Read the model definition and answer for the solid it produces. Units are mm, in the model's axes. Face numbers are marked on the shaded views. A direction names the side the tool comes from. Coordinates: 2 decimals unless noted, no trailing zeros. Order: outer loops, then holes, each group sorted by start corner. A loop starts at its lowest first (then second) coordinate and runs counter-clockwise, first axis right, second up.
Autodesk Fusion 360 part; units mm, degrees
box "BoxPrimitive1" add length 65 width 15 height 4 placed x (0, 0, -1) y (-1, 0, 0) z (0, 1, 0) at (0, 0, 0)
sketch "Sketch2" plane through (0, 4, 0) normal (0, 1, 0) x (-1, 0, 0)
  line L0 (0, -65) -> (15, -65)
  line L1 (15, -65) -> (15, 0)
  line L2 (15, 0) -> (0, 0)
  line L3 (0, 0) -> (0, -65)
  line L4 (15, -65) -> (0, -65)
  line L5 (0, -65) -> (0, -61)
  line L6 (0, -61) -> (15, -61)
  line L7 (15, -61) -> (15, -65)
  dimension "d6" = 4
extrude "Extrude1" add sketch "Sketch2" along normal blind 35 contours L0 L1 L3 L4 L5 L6 L7
chamfer "Chamfer1" distance 9 angle 45 1 edges at (-7.5, 4, -61)
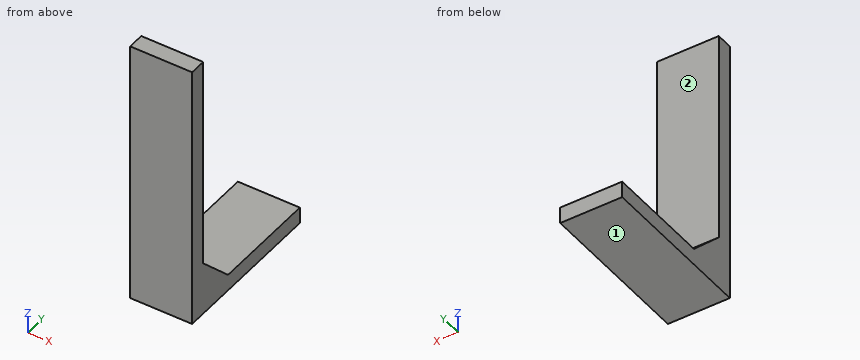
1) A cutting plane is placed at C-C, the plane y = 6.5. Determine the outline of the cut face in (x, z), and give its area (4 significant figures).
A:
outline: (-15, -65) - (0, -65) - (0, -54.5) - (-15, -54.5) - close
area: 157.5 mm2
2) Straight lines are drawn through the part: line 1 (Y direction, x = -7.75, z = -44.5); line 2 (Z direction, x = -11, y = 36.5); line 3 (Y direction, x = -7.75, z = -60). For each, find the intervals that lie inside material, in ascending order.
A:
line 1: y = 0 to 4
line 2: z = -65 to -61
line 3: y = 0 to 12
3) A cutting plane is placed at A-A, the plane x = -3.5. Determine the outline of the cut face in (y, z), and give its area (4 significant figures).
A:
outline: (0, -65) - (39, -65) - (39, -61) - (13, -61) - (4, -52) - (4, 0) - (0, 0) - close
area: 440.5 mm2
4) Which of the six approach directions +Z, -Z, +X, -X, +Y, -Y give full straight-line access (tool end or side, diameter ignored) to the marked faces 1 and 2?
A:
face 1: -Z, +X, -X, +Y, -Y
face 2: +Z, +X, -X, +Y
5) Flat-ended cylindrical pins translate along their axes: pin 1 Ø8 at (x, y) = (-3, 31.5) entering from +Z; pin 2 Ø3 at (x, z) = (-8.5, -30.5) entering from +Y; pin 3 Ø3 at (x, z) = (-1.5, -57) entering from -Y; pin 4 Ø10 at (y, z) = (12.5, -22.5) entering from +X. Find the tip coordinate at first contact, or state that the pin passes through.
A:
pin 1: stops at z = -61
pin 2: stops at y = 4
pin 3: stops at y = 0
pin 4: passes through
6) A cutting plane is placed at B-B, the plane z = -46. Determine the outline of the cut face in (x, y), and give its area (3 significant figures).
A:
outline: (-15, 0) - (0, 0) - (0, 4) - (-15, 4) - close
area: 60.0 mm2
